from build123d import *

# Parameters (mm, degrees)
SKETCH1_W           = 39.6875
SKETCH1_H           = 39.6875
SKETCH1_W_2         = 36.5125
SKETCH1_H_2         = 36.5125
BOSS_EXTRUDE1_DEPTH = 305.59375
FILLET1_R           = 1.27
FILLET2_R           = 0.635
SKETCH2_R           = 7.9375
BOSS_EXTRUDE2_DEPTH = 92.075
CHAMFER1_SIZE       = 2.54


with BuildPart() as part:
    # Sketch1 → Boss-Extrude1 (new, symmetric)
    with BuildSketch(Plane.XY):
        Rectangle(SKETCH1_W, SKETCH1_H)
        Rectangle(SKETCH1_W_2, SKETCH1_H_2, mode=Mode.SUBTRACT)
    extrude(amount=BOSS_EXTRUDE1_DEPTH, both=True)

    # Fillet1
    fillet1_edges = [part.edges().sort_by_distance(p)[0] for p in [
        (-19.84375, 19.84375, 0),
        (19.84375, 19.84375, 0),
        (19.84375, -19.84375, 0),
        (-19.84375, -19.84375, 0),
    ]]
    fillet(fillet1_edges, radius=FILLET1_R)

    # Fillet2
    fillet2_edges = [part.edges().sort_by_distance(p)[0] for p in [
        (18.25625, -18.25625, 0),
        (18.25625, 18.25625, 0),
        (-18.25625, 18.25625, 0),
        (-18.25625, -18.25625, 0),
    ]]
    fillet(fillet2_edges, radius=FILLET2_R)

    # Sketch2 → Boss-Extrude2 (add, symmetric)
    with BuildSketch(Plane(origin=(0, 0, 0), x_dir=(0, 0, -1), z_dir=(1, 0, 0))):
        with Locations(Location((0, 0, 0), (0, 0, 270))):
            Circle(SKETCH2_R)
    extrude(amount=BOSS_EXTRUDE2_DEPTH, both=True)

    # Chamfer1
    chamfer1_edges = [part.edges().sort_by_distance(p)[0] for p in [
        (19.84375, 7.9375, 0),
        (-19.84375, 7.9375, 0),
    ]]
    chamfer(chamfer1_edges, length=CHAMFER1_SIZE)


solid = part.part
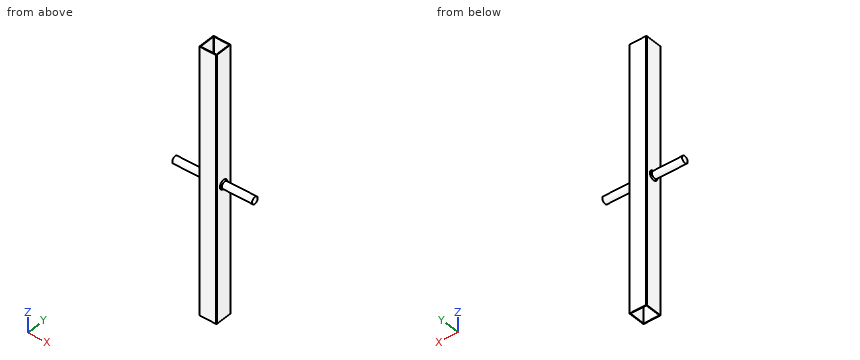
Here's how the part is built. I have some questions about the finished solid (model axes, mm). Give positions to 0.01 mm unless a question says otherwise; leave off trailing zeros. Loops run counter-clockwise (first coordinate to the right, second up) from the corner with the lowest first, then second, coordinate; pieces in that order, holes last. Notation, with made-up numbers: (-20.5, -19) -> (18.5, -19) arc R28 cw to (18.5, 1) -> close; hole circle Ø7 at (37, -3). An arc over 180 degrees is marked (long way). Answer as a JSON object with one key per item and string values. Group by question number.
Item 1: Imagine slicing it at D-D on y = 0. Write out the boundary of the cut face in (x, z) (1 decimal).
Item 2: Imagine slicing it at B-B on z = -153.5. Write out the boundary of the cut face in (x, y) (3 decimals).
Item 3: Imagine slicing it at A-A on x = 4. Write out the boundary of the cut face in (y, z) (1 decimal).
Item 4: Imagine slicing it at C-C on z = 0. Give the number of separate pieces and of enclosed holes in the cut face, then the cut area to 3 significant figures.
Item 5: I need wall thicknesses on L1, parallel to X at y = -8, z = 199; L2, parallel to X at y = 18, z = 233. Which ranges of each line are inside material? Lowest first, please.
Item 6: Will these pins go through, and if not, where does the flat tip stop? pin 1 (1.5 mm diameter, centred on y = 11.5, z = -29.5, fed in from -X); pin 2 (1 mm diameter, centred on x = 64.5, y = 3.5, fed in from -Z); pin 3 (6 mm diameter, centred on y = 15, z = 136.5, fed in from +X).
Answer list:
{
 "1": {"outline": "(-92.1, -7.9) -> (-22.4, -7.9) -> (-19.8, -10.5) -> (-19.8, -305.6) -> (-18.3, -305.6) -> (-18.3, -7.9) -> (18.3, -7.9) -> (18.3, -305.6) -> (19.8, -305.6) -> (19.8, -10.5) -> (22.4, -7.9) -> (92.1, -7.9) -> (92.1, 7.9) -> (22.4, 7.9) -> (19.8, 10.5) -> (19.8, 305.6) -> (18.3, 305.6) -> (18.3, 7.9) -> (-18.3, 7.9) -> (-18.3, 305.6) -> (-19.8, 305.6) -> (-19.8, 10.5) -> (-22.4, 7.9) -> (-92.1, 7.9) -> close"},
 "2": {"outline": "(-19.844, -18.574) arc R1.27 ccw to (-18.574, -19.844) -> (18.574, -19.844) arc R1.27 ccw to (19.844, -18.574) -> (19.844, 18.574) arc R1.27 ccw to (18.574, 19.844) -> (-18.574, 19.844) arc R1.27 ccw to (-19.844, 18.574) -> close; hole (-18.256, -17.621) arc R0.635 ccw to (-17.621, -18.256) -> (17.621, -18.256) arc R0.635 ccw to (18.256, -17.621) -> (18.256, 17.621) arc R0.635 ccw to (17.621, 18.256) -> (-17.621, 18.256) arc R0.635 ccw to (-18.256, 17.621) -> close"},
 "3": {"outline": "(-19.8, -305.6) -> (-18.3, -305.6) -> (-18.3, 305.6) -> (-19.8, 305.6) -> close; circle Ø15.9 at (0, 0); (18.3, -305.6) -> (19.8, -305.6) -> (19.8, 305.6) -> (18.3, 305.6) -> close"},
 "4": {"separate pieces": "1", "enclosed holes": "2", "area": "3,130 mm2"},
 "5": {"L1": "x = -19.84 to -18.26, 18.26 to 19.84", "L2": "x = -19.84 to -18.13, 18.13 to 19.84"},
 "6": {"pin 1": "stops at x = -19.84", "pin 2": "stops at z = -7.35", "pin 3": "stops at x = 19.84"}
}
